from build123d import *

# Parameters (mm, degrees)
SKETCH1_R           = 2
SKETCH1_R_2         = 3
BOSS_EXTRUDE1_DEPTH = 9.5
SKETCH2_W           = 173.341634435
SKETCH2_H           = 7
CUT_EXTRUDE1_DEPTH  = 2


with BuildPart() as part:
    # Sketch1 → Boss-Extrude1 (new body)
    with BuildSketch(Plane(origin=(0, 0, 0), x_dir=(1, 0, 0), z_dir=(0, 1, 0))):
        with BuildLine():
            Line((97, 16), (97, 24))
            ThreePointArc((97, 24), (90, 31), (83, 24))
            Line((83, 24), (83, 16))
            Line((83, 16), (-10, 16))
            ThreePointArc((-10, 16), (-18, 8), (-10, 0))
            Line((-10, 0), (190, 0))
            ThreePointArc((190, 0), (198, 8), (190, 16))
            Line((190, 16), (97, 16))
        make_face()
        with Locations(Location((90, 24, 0), (0, 0, 270))):
            Circle(SKETCH1_R, mode=Mode.SUBTRACT)
        with Locations(Location((-10, 8, 0), (0, 0, 270))):
            Circle(SKETCH1_R_2, mode=Mode.SUBTRACT)
        with Locations(Location((190, 8, 0), (0, 0, 270))):
            Circle(SKETCH1_R, mode=Mode.SUBTRACT)
    extrude(amount=BOSS_EXTRUDE1_DEPTH)

    # Sketch2 → Cut-Extrude1 (cut)
    with BuildSketch(Plane(origin=(0, 9.5, 0), x_dir=(1, 0, 0), z_dir=(0, 1, 0))):
        with Locations((89.670817218, 8)):
            Rectangle(SKETCH2_W, SKETCH2_H)
    extrude(amount=-CUT_EXTRUDE1_DEPTH, mode=Mode.SUBTRACT)


solid = part.part
Can you work these out from the model? Positions are in its coordinate system, mm. A direction names the side the tool comes from. Give positions to 0.01 mm unless a question says otherwise; leave off trailing zeros. Order: outer loops, then holes, each group sorted by start corner. A loop starts at its lowest first (then second) coordinate and runs counter-clockwise, first axis right, second up. Notation, with made-up numbers: (48, 54) - (70, 54) arc R33 cw to (70, 87) - close; hole circle Ø9 at (76.25, -38). An arc over 180 degrees is marked (long way). Write each question's results on one line, items separated by ' | '.
1) Suppose I cut it at A-A, the plane x = 90. Write out the boundary of the cut face in (y, z), then the cut area to 4 significant figures.
Final values:
outline: (0, -31) - (9.5, -31) - (9.5, -26) - (0, -26) - close; (0, -22) - (9.5, -22) - (9.5, -11.5) - (7.5, -11.5) - (7.5, -4.5) - (9.5, -4.5) - (9.5, 0) - (0, 0) - close | area: 242.5 mm^2
2) Please list where these lines run through material, in increasing order: line 1 along X through (y, z) = (7.25, -8); line 2 along Z through (x, y) = (22, 6.75); line 3 along X through (y, z) = (6.5, -24). Write a range as [from, to].
Final values:
line 1: x = [-18, -13], [-7, 188], [192, 198] | line 2: z = [-16, 0] | line 3: x = [83, 88], [92, 97]
3) I'm going to push flat-ended pins straight in: pin 1 Ø5 at (x, y) = (21, 6) entering from -Z; pin 2 Ø1.6 at (y, z) = (8.5, -9.5) entering from -X; pin 3 Ø3 at (y, z) = (5, -16) entering from +X; pin 4 Ø2 at (y, z) = (8.5, -9) entering from +X. Where does each tip first touch, or does it pass through?
Final values:
pin 1: stops at z = -16 | pin 2: stops at x = -17.97 | pin 3: stops at x = 194.66 | pin 4: stops at x = 198
4) Suppose I cut it at B-B, the plane z = -8. Write out the boundary of the cut face in (x, y), then the cut area to 3 significant figures.
Final values:
outline: (-18, 0) - (-13, 0) - (-13, 9.5) - (-18, 9.5) - close; (-7, 0) - (188, 0) - (188, 9.5) - (176.34, 9.5) - (176.34, 7.5) - (3, 7.5) - (3, 9.5) - (-7, 9.5) - close; (192, 0) - (198, 0) - (198, 9.5) - (192, 9.5) - close | area: 1,610 mm^2
5) Suppose I cut it at D-D, the plane x = 144. Write out the boundary of the cut face in (y, z).
Final values:
outline: (0, -16) - (9.5, -16) - (9.5, -11.5) - (7.5, -11.5) - (7.5, -4.5) - (9.5, -4.5) - (9.5, 0) - (0, 0) - close
6) On a 3-axis mill with a long thin cutter (end or side, diameter ignored), from which of +Z, -Z, +X, -X, +Y, -Y can I reach the whole of each face in a straight line? I mean faces 1 (the face through (144, 5, -16)), 2 (the face through (37, 5, -16)), 3 (the face through (89, 5, 0)), 4 (the face through (90, 5, -31)), 5 (the face through (88, 7.5, -8)). Say none if no direction works.
Final values:
face 1: -Z, +X, +Y, -Y | face 2: -Z, -X, +Y, -Y | face 3: +Z, +X, -X, +Y, -Y | face 4: -Z, +Y, -Y | face 5: +Y
7) If we mould it in two halves opening along X, with no side actions, what happens to faces 6 (the face through (97, 5, -20)), 7 (the face through (-9.1, 4.68, -5.14)), 8 (the face through (88, 9.5, -12)), 9 (the face through (92, 5, -24))? For each: pulls with the +X half, pulls with the -X half, needs draft (parallel to the pull), parting line crosses it, or undercut.
Final values:
face 6: pulls with the +X half | face 7: undercut | face 8: needs draft | face 9: undercut
8) Suppose I cut it at C-C, the plane y = 4.75. Write out the boundary of the cut face in (x, z), then the cut area to 3 significant figures.
Final values:
outline: (-10, -16) - (83, -16) - (83, -24) arc R7 ccw to (97, -24) - (97, -16) - (190, -16) arc R8 ccw to (190, 0) - (-10, 0) arc R8 ccw to start; hole circle Ø6 at (-10, -8); hole circle Ø4 at (90, -24); hole circle Ø4 at (190, -8) | area: 3,540 mm^2
